Verification items for the finished model (mm, model axes). A direction names the side the tool comes from. Give positions to 0.01 mm unless a question says otherwise; leave off trailing zeros. Loops run counter-clockwise (first coordinate to the right, second up) from the corner with the lowest first, then second, coordinate; pieces in that order, holes last. Notation, with made-up numbers: (82.5, 10.5) - (126.5, 10.5) arc R32 ccw to (126.5, 36.5) - close; hole circle Ø10 at (0.25, 31). An arc over 180 degrees is marked (long way). Answer in a Markdown table with one row per item.
```python
from build123d import *

# Parameters (mm, degrees)
SKETCH2_W              = 242.645613954
SKETCH2_H              = 231.138030636
CUT_IN_HALF_DEPTH      = 165.544826719
SKETCH3_R              = 11
BALLBEARINGHOLE_DEPTH  = 165.544826719
SKETCH4_R              = 31.202879122
SUPPORTFORHOLE_DEPTH   = 4
F_2NDBEARINGHOLE_START = -7
SKETCH5_R              = 11
F_2NDBEARINGHOLE_DEPTH = 7
SKETCH6_R              = 4.5
INSIDEHOLE_DEPTH       = 161.277134988


with BuildPart() as part:
    # Half Circle → Sphere Revolve (revolve)
    with BuildSketch(Plane.XY):
        with BuildLine():
            Line((0, 85), (0, 95))
            ThreePointArc((0, 95), (-95, 0), (0, -95))
            Line((0, -95), (0, -85))
            ThreePointArc((0, -85), (-85, 0), (0, 85))
        make_face()
    revolve(axis=Axis((0, 85, 0), (0, 1, 0)))

    # Sketch2 → Cut in Half (cut, through all)
    with BuildSketch(Plane(origin=(0, 0, 0), x_dir=(1, 0, 0), z_dir=(0, 1, 0))):
        Rectangle(SKETCH2_W, SKETCH2_H)
    extrude(amount=-CUT_IN_HALF_DEPTH, mode=Mode.SUBTRACT)

    # Sketch3 → BallBearingHole (cut, through all)
    with BuildSketch(Plane(origin=(0, 0, 0), x_dir=(1, 0, 0), z_dir=(0, 1, 0))):
        with Locations(Location((0, 0, 0), (0, 0, 90))):
            Circle(SKETCH3_R)
    extrude(amount=BALLBEARINGHOLE_DEPTH, mode=Mode.SUBTRACT)

    # Sketch4 → SupportForHole (add)
    with BuildSketch(Plane(origin=(0, 84.4, 0), x_dir=(1, 0, 0), z_dir=(0, 1, 0))):
        Circle(SKETCH4_R)
    extrude(amount=SUPPORTFORHOLE_DEPTH)

    # Sketch5 → 2ndBearingHole (cut)
    with BuildSketch(Plane(origin=(0, 94.4, 0), x_dir=(1, 0, 0), z_dir=(0, 1, 0)).offset(F_2NDBEARINGHOLE_START)):
        with Locations(Location((0, 0, 0), (0, 0, 90))):
            Circle(SKETCH5_R)
    extrude(amount=F_2NDBEARINGHOLE_DEPTH, mode=Mode.SUBTRACT)

    # Sketch6 → InsideHole (cut, through all)
    with BuildSketch(Plane(origin=(0, 87.4, 0), x_dir=(1, 0, 0), z_dir=(0, 1, 0))):
        with Locations(Location((0, 0, 0), (0, 0, 270))):
            Circle(SKETCH6_R)
    extrude(amount=-INSIDEHOLE_DEPTH, mode=Mode.SUBTRACT)


solid = part.part
```
Q1. Tool access check on faces 4 (the face through (-9.275, 90.832, -5.914)), 5 (the face through (0, 84.4, 5)). Record the directions out of +Z, -Z, +X, -X, +Y, -Y that give a thin tool (end or side, any length) a straight path to the whole face; none if there is none.
Completed:
| item | result |
|---|---|
| face 4 | +Y |
| face 5 | -Y |
Q2. Sectioned sample at A-A (x = 0). Record the cut outline in (y, z).
Completed:
| item | result |
|---|---|
| outline | (0, -95) arc R95 ccw to (94.36, -11) - (87.4, -11) - (87.4, -4.5) - (84.4, -4.5) - (84.4, -11) - (84.29, -11) arc R85 cw to (0, -85) - close; (0, 85) arc R85 cw to (84.29, 11) - (84.4, 11) - (84.4, 4.5) - (87.4, 4.5) - (87.4, 11) - (94.36, 11) arc R95 ccw to (0, 95) - close |
Q3. Go/stop test with flat-tipped pins: P1, Ø1, axis at x = -40.5, z = -60.5, coming from the +Y side; P2, Ø4, axis at x = -20.5, z = 69, coming from the +Y side; P3, Ø8, axis at x = 36.5, y = 46, coming from the -Z side; P4, Ø8, axis at x = 0, z = 0, coming from the -Y side. Record where each tip stops, or that it passes through.
Completed:
| item | result |
|---|---|
| P1 | y = 61.62 |
| P2 | y = 64.25 |
| P3 | z = -77.66 |
| P4 | through |
Q4. Sectioned sample at B-B (z = 0). Record the cut outline in (x, y).
Completed:
| item | result |
|---|---|
| outline | (-95, 0) - (-85, 0) arc R85 cw to (-11, 84.29) - (-11, 84.4) - (-4.5, 84.4) - (-4.5, 87.4) - (-11, 87.4) - (-11, 94.36) arc R95 ccw to start; (4.5, 84.4) - (11, 84.4) - (11, 84.29) arc R85 cw to (85, 0) - (95, 0) arc R95 ccw to (11, 94.36) - (11, 87.4) - (4.5, 87.4) - close |
Q5. Draft check along Y on faces 1 (the face through (5, 87.4, 0)), 2 (the face through (-71, 0, 49)), 3 (the face through (1.352, 85.921, 4.292)). Enter one of: +Y half, -Y half, draft (parallel to the pull), parting line (faces both ways), or undercut.
Completed:
| item | result |
|---|---|
| face 1 | +Y half |
| face 2 | -Y half |
| face 3 | draft |
Q6. Sectioned sample at C-C (x = 66.5). Record the cut outline in (y, z).
Completed:
| item | result |
|---|---|
| outline | (0, -67.84) arc R67.84 ccw to (0, 67.84) - (0, 52.94) arc R52.94 cw to (0, -52.94) - close |
Q7. Sectioned sample at D-D (y = 69.5). Record the cut outline in (x, z).
Completed:
| item | result |
|---|---|
| outline | circle Ø129.53 at (0, 0); hole circle Ø97.87 at (0, 0) |
Q8. Thickness scan on line 1 (X direction, y = 46.5, z = 34); line 2 (X direction, y = 85.3, z = 0); line 3 (Z direction, x = -59.5, y = 22). Record the ranges inside material, lowest first.
Completed:
| item | result |
|---|---|
| line 1 | -75.54 to -62.5, 62.5 to 75.54 |
| line 2 | -41.82 to -4.5, 4.5 to 41.82 |
| line 3 | -70.72 to -56.58, 56.58 to 70.72 |
